Verification items for the finished model (mm, model axes). A direction names the side the tool comes from. Coordinates: 2 decimals unless noted, no trailing zeros. Loops run counter-clockwise (first coordinate to the right, second up) from the corner with the lowest first, then second, coordinate; pieces in that order, holes last. Notation, with made-up numbers: M -26.75,15 L 14.25,15 A31 ccw 14.25,53 Z; hole C 24.5,72 d7. An arc over 180 degrees is marked long. Write item = value, one per line. Start each with the question number.
```python
from build123d import *

# Parameters (mm, degrees)
SKETCH2_R           = 35
BOSS_EXTRUDE1_DEPTH = 6
SKETCH8_W           = 70
SKETCH8_H           = 70
BOSS_EXTRUDE3_DEPTH = 6
SKETCH3_R           = 0.8
CUT_EXTRUDE1_DEPTH  = 6
SKETCH4_R           = 0.6
CUT_EXTRUDE2_DEPTH  = 6
SKETCH5_W           = 3
SKETCH5_H           = 10
BOSS_EXTRUDE2_DEPTH = 10
CUT_EXTRUDE3_DEPTH  = 84.408632647
SKETCH7_R           = 1.5
CUT_EXTRUDE4_DEPTH  = 84.408632647


with BuildPart() as part:
    # Sketch2 → Boss-Extrude1 (new body)
    with BuildSketch(Plane.XY):
        Circle(SKETCH2_R)
    extrude(amount=BOSS_EXTRUDE1_DEPTH)

    # Sketch8 → Boss-Extrude3 (add)
    with BuildSketch(Plane(origin=(0, 0, 0), x_dir=(-1, 0, 0), z_dir=(0, 0, -1))):
        with Locations((35, 0)):
            Rectangle(SKETCH8_W, SKETCH8_H)
    extrude(amount=-BOSS_EXTRUDE3_DEPTH)

    # Sketch3 → Cut-Extrude1 (cut)
    with BuildSketch(Plane.XY.offset(6)):
        with Locations((0, 30.914278185)):
            Circle(SKETCH3_R)
        with Locations((26.846787517, -15.585721815)):
            Circle(SKETCH3_R)
        with Locations((-26.846787517, -15.585721815)):
            Circle(SKETCH3_R)
    extrude(amount=-CUT_EXTRUDE1_DEPTH, mode=Mode.SUBTRACT)

    # Sketch4 → Cut-Extrude2 (cut)
    with BuildSketch(Plane.XY.offset(6)):
        Circle(SKETCH4_R)
    extrude(amount=-CUT_EXTRUDE2_DEPTH, mode=Mode.SUBTRACT)

    # Sketch5 → Boss-Extrude2 (add)
    with BuildSketch(Plane.XY.offset(6)):
        with Locations((2.5, 0)):
            Rectangle(SKETCH5_W, SKETCH5_H)
        with Locations((-2.5, 0)):
            Rectangle(SKETCH5_W, SKETCH5_H)
    extrude(amount=BOSS_EXTRUDE2_DEPTH)

    # Sketch6 → Cut-Extrude3 (cut, through all)
    with BuildSketch(Plane(origin=(4, 0, 0), x_dir=(0, 0, -1), z_dir=(1, 0, 0))):
        with BuildLine():
            ThreePointArc((-16, 0), (-14.535533906, 3.535533906), (-11, 5))
            Line((-11, 5), (-16, 5))
            Line((-16, 5), (-16, 0))
        make_face()
        with BuildLine():
            ThreePointArc((-11, -5), (-14.535533906, -3.535533906), (-16, 0))
            Line((-16, 0), (-16, -5))
            Line((-16, -5), (-11, -5))
        make_face()
    extrude(amount=-CUT_EXTRUDE3_DEPTH, mode=Mode.SUBTRACT)

    # Sketch7 → Cut-Extrude4 (cut, through all)
    with BuildSketch(Plane(origin=(4, 0, 0), x_dir=(0, 0, -1), z_dir=(1, 0, 0))):
        with Locations(Location((-11, 2.8, 0), (0, 0, 90))):
            Circle(SKETCH7_R)
        with Locations(Location((-11, -2.8, 0), (0, 0, 90))):
            Circle(SKETCH7_R)
    extrude(amount=-CUT_EXTRUDE4_DEPTH, mode=Mode.SUBTRACT)


solid = part.part
```
Q1. Sectioned sample at D-D on y = -25. Record the cut outline in (x, z), plus the area to 3 significant figures.
Q2. Sectioned sample at A-A on z = 3.75. Record the cut outline in (x, y), plus the area to 3 significant figures.
Q3. Sectioned sample at B-B on y = 2.8. Record the cut outline in (x, z), plus the area to 3 significant figures.
Q4. Mould release check, pull along Y, two halves, no side actions. Record for faces 5 (the face through (-3, -5, 8)), 6 (the face through (-2.48, -4.3, 11.07)), 7 (the face through (4, 0, 11)): +Y half, -Y half, draft (parallel to the pull), parting line (faces both ways), or undercut.
Q5. Set-up check for faces 1 (the face through (2, -5, 8)), 2 (the face through (-4, 0, 11)), 3 (the face through (-3, 5, 8)), 4 (the face through (-1, 0, 11)): record each of +Z, -Z, +X, -X, +Y, -Y from which the full face is reachable in a straight line by a thin tool's end or side.
Q6. Gauge pin test, flat ends, axial feed: pin 1 (3 mm diameter, centred on y = 1.5, z = 12, fed in from -X); pin 2 (6 mm diameter, centred on x = 16, y = 8, fed in from +Z); pin 3 (0.9 mm diameter, centred on x = 3, z = 8.5, fed in from +Y). Record the tip position at first contact, or that the pin passes through.
Q7. Scan lines: L1, parallel to Y at x = 0, z = 2.05; L2, parallel to X at y = -2.5, z = 7.5; L3, parallel to Z at x = -23.5, y = -26.5. Record each from-to range of solid material in increasing order. Write a range as [from, to].
Q8. Sectioned sample at C-C on x = -55.5. Record the cut outline in (y, z).
Solutions:
q1.outline = M -70,0 L 24.49,0 L 24.49,6 L -70,6 Z
q1.area = 567 mm²
q2.outline = M -70,-35 L 0,-35 A35 ccw 0,35 L -70,35 Z; hole C -26.85,-15.59 d1.6; hole C 0,30.91 d1.6; hole C 0,0 d1.2; hole C 26.85,-15.59 d1.6
q2.area = 6,820 mm²
q3.outline = M -70,0 L 34.89,0 L 34.89,6 L 4,6 L 4,9.5 L 1,9.5 L 1,6 L -1,6 L -1,9.5 L -4,9.5 L -4,6 L -70,6 Z; M -4,12.5 L -1,12.5 L -1,15.14 L -4,15.14 Z; M 1,12.5 L 4,12.5 L 4,15.14 L 1,15.14 Z
q3.area = 666 mm²
q4.face_5 = -Y half
q4.face_6 = undercut
q4.face_7 = draft
q5.face_1 = +Z, +X, -X, -Y
q5.face_2 = +Z, -X, +Y, -Y
q5.face_3 = +Z, +X, -X, +Y
q5.face_4 = +Z, +Y, -Y
q6.pin_1 = -4
q6.pin_2 = 6
q6.pin_3 = 5
q7.L1 = [-35, -0.6], [0.6, 30.11], [31.71, 35]
q7.L2 = [-4, -1], [1, 4]
q7.L3 = [0, 6]
q8.outline = M -35,0 L 35,0 L 35,6 L -35,6 Z
